from build123d import *

# Parameters (mm, degrees)
CYLINDER010_R     = 0.5
CYLINDER010_DEPTH = 2
ARRAY_X_COUNT     = 2
ARRAY_X_PITCH     = 15.24
ARRAY_Y_COUNT     = 7
ARRAY_Y_PITCH     = 2.54
BOX028_W          = 17.78
BOX028_H          = 20.9982
BOX028_DEPTH      = 1.2
FILLET009_R       = 2.03


with BuildPart() as obj1:
    # Cylinder010 → Cylinder010 (new body)
    with BuildSketch(Plane(origin=(-7.62, -7.62, 0), x_dir=(1, 0, 0), z_dir=(0, 0, 1))):
        Circle(CYLINDER010_R)
    extrude(amount=CYLINDER010_DEPTH)

    # Array X: obj1_2


with BuildPart() as obj1_1:
    add(obj1.part)
    with Locations(*[(i * ARRAY_X_PITCH, 0, 0) for i in range(1, ARRAY_X_COUNT)]):
        add(obj1.part)

    # Array Y: obj1 ×7


with BuildPart() as obj1_2:
    add(obj1_1.part)
    with Locations(*[(0, i * ARRAY_Y_PITCH, 0) for i in range(1, ARRAY_Y_COUNT)]):
        add(obj1_1.part)


with BuildPart() as obj2:
    # Box028 → Box028 (new body)
    with BuildSketch(Plane(origin=(-8.89, -10.508, 0), x_dir=(1, 0, 0), z_dir=(0, 0, 1))):
        with Locations((8.89, 10.4991)):
            Rectangle(BOX028_W, BOX028_H)
    extrude(amount=BOX028_DEPTH)

    # Fillet009
    fillet009_edges = [obj2.edges().sort_by_distance(p)[0] for p in [
        (-8.89, -10.508, 0.6),
        (-8.89, 10.4902, 0.6),
        (8.89, -10.508, 0.6),
        (8.89, 10.4902, 0.6),
    ]]
    fillet(fillet009_edges, radius=FILLET009_R)

    # Cut004: cut obj1
    add(obj1_2.part, mode=Mode.SUBTRACT)


solid = obj2.part
CAD build for the part. Positions are in the model's coordinates, mm. Coordinates: 2 decimals unless noted, no trailing zeros. Loops run counter-clockwise (first coordinate to the right, second up) from the corner with the lowest first, then second, coordinate; pieces in that order, holes last. Notation, with made-up numbers: (24, 66.25) -> (75, 66.25) arc R14 cw to (75, 86.25) -> close; hole circle Ø6 at (80.25, 45). An arc over 180 degrees is marked (long way). One line per item, written item: value.
1. Drill centre lines: line 1 (X direction, y = -5.08, z = 0.35); line 2 (X direction, y = -0.25, z = 0.4); line 3 (X direction, y = 9.75, z = 0.4). Where is each one in solid material? Low to high. Write a range as [from, to].
Answers:
line 1: x = [-8.89, -8.12], [-7.12, 7.12], [8.12, 8.89]
line 2: x = [-8.89, -8.05], [-7.19, 7.19], [8.05, 8.89]
line 3: x = [-8.43, 8.43]
2. Pull direction Y, two halves, no side cores. Call faces 1 (the face through (0, -10.508, 1)), 2 (the face through (0, 0, 1.2)), 3 (the face through (8.1, -2.4, 0.6)): pulls with the +Y half, pulls with the -Y half, needs draft (parallel to the pull), parting line crosses it, or undercut.
Answers:
face 1: pulls with the -Y half
face 2: needs draft
face 3: undercut
3. Slice it at A-A on y = 0. Write the cut outline in (x, z), and give its area (3 significant figures).
Answers:
outline: (-8.89, 0) -> (-8.12, 0) -> (-8.12, 1.2) -> (-8.89, 1.2) -> close; (-7.12, 0) -> (7.12, 0) -> (7.12, 1.2) -> (-7.12, 1.2) -> close; (8.12, 0) -> (8.89, 0) -> (8.89, 1.2) -> (8.12, 1.2) -> close
area: 18.9 mm^2
4. Slice it at B-B on z = 0.85. Give the number of separate pieces and of enclosed holes in the cut face, and give its area (3 significant figures).
Answers:
separate pieces: 1
enclosed holes: 14
area: 359 mm^2
